Input: part model. Units: mm. Frame: model coordinates. Coordinates: 2 decimals unless noted, no trailing zeros. Order: outer loops, then holes, each group sorted by start corner. A loop starts at its lowest first (then second) coordinate and runs counter-clockwise, first axis right, second up. Notation, with made-up numbers: (70, 18) -> (94, 18) arc R15 ccw to (94, 25) -> close; hole circle Ø3 at (31, -6). An arc over 180 degrees is marked (long way). Use one line per item in the form item = value. Start each with the question number.
1) Pin query (flat end, axial travel): pin 1 (2.5 mm diameter, centred on y = 160.5, z = 3, fed in from +X) (3 decimals); pin 2 (1.5 mm diameter, centred on y = 41, z = 3, fed in from -X) (3 decimals); pin 3 (1.4 mm diameter, centred on x = 116, z = 3, fed in from +Y). Return the tip coordinate at first contact, or that it passes through.
2) Section query B-B on x = 100. Output: boundary loops of the cut face in (y, z), then the cut area to 3 significant figures.
3) Section query A-A on y = 130. Output: boundary loops of the cut face in (x, z).
4) Ray query, line 1 along X through (y, z) = (9.5, 0.4); line 2 along Y through (x, z) = (19, 0.35); line 3 along Y through (x, z) = (103, 1.05). Return the intervals inside material, ascending.
from build123d import *

# Parameters (mm, degrees)
BOSS_EXTRUDE1_DEPTH = 4.826
CUT_EXTRUDE1_DEPTH  = 283.027055929
SKETCH3_R           = 23.114
CUT_EXTRUDE2_DEPTH  = 4.826
SKETCH4_W           = 20.32
SKETCH4_H           = 4.617249963
CUT_EXTRUDE3_DEPTH  = 283.027055929
SKETCH5_W           = 20.32
SKETCH5_H           = 4.826
CUT_EXTRUDE4_DEPTH  = 283.027055929


with BuildPart() as part:
    # Sketch1 → Boss-Extrude1 (new body)
    with BuildSketch(Plane.XY):
        Polygon((228.6, 165.1), (0, 165.1), (82.55, 0), (146.05, 0), align=None)
    extrude(amount=BOSS_EXTRUDE1_DEPTH)

    # Sketch2 → Cut-Extrude1 (cut, through all)
    with BuildSketch(Plane.XY.offset(4.826)):
        Polygon((20.097936797, 124.904126406), (24.414442421, 127.062379218), (35.002974022, 105.885316015), (30.686468399, 103.727063203), align=None)
        Polygon((41.275, 82.55), (45.591505624, 84.708252812), (56.180037225, 63.531189609), (51.863531601, 61.372936797), align=None)
        Polygon((62.452063203, 40.195873594), (66.768568827, 42.354126406), (77.357100428, 21.177063203), (73.040594804, 19.018810391), align=None)
        Polygon((155.559405196, 19.018810391), (166.147936797, 40.195873594), (161.831431173, 42.354126406), (151.242899572, 21.177063203), align=None)
        Polygon((176.736468399, 61.372936797), (187.325, 82.55), (183.008494376, 84.708252812), (172.419962775, 63.531189609), align=None)
        Polygon((197.913531601, 103.727063203), (208.502063203, 124.904126406), (204.185557579, 127.062379218), (193.597025978, 105.885316015), align=None)
    extrude(amount=-CUT_EXTRUDE1_DEPTH, mode=Mode.SUBTRACT)

    # Sketch3 → Cut-Extrude2 (cut)
    with BuildSketch(Plane.XY.offset(4.826)):
        with Locations((114.3, -7.62)):
            Circle(SKETCH3_R)
    extrude(amount=-CUT_EXTRUDE2_DEPTH, mode=Mode.SUBTRACT)

    # Sketch4 → Cut-Extrude3 (cut, through all)
    with BuildSketch(Plane.XY.offset(4.826)):
        with Locations((154.974498273, 165.599419735)):
            Rectangle(SKETCH4_W, SKETCH4_H)
        with Locations((114.334498273, 165.599419735)):
            Rectangle(SKETCH4_W, SKETCH4_H)
        with Locations((73.694498273, 165.599419735)):
            Rectangle(SKETCH4_W, SKETCH4_H)
    extrude(amount=-CUT_EXTRUDE3_DEPTH, mode=Mode.SUBTRACT)

    # Sketch5 → Cut-Extrude4 (cut, through all)
    with BuildSketch(Plane.XY.offset(4.826)):
        with Locations((154.974498273, 160.877794753)):
            Rectangle(SKETCH5_W, SKETCH5_H)
        with Locations((114.334498273, 160.877794753)):
            Rectangle(SKETCH5_W, SKETCH5_H)
        with Locations((73.694498273, 160.877794753)):
            Rectangle(SKETCH5_W, SKETCH5_H)
    extrude(amount=-CUT_EXTRUDE4_DEPTH, mode=Mode.SUBTRACT)


solid = part.part
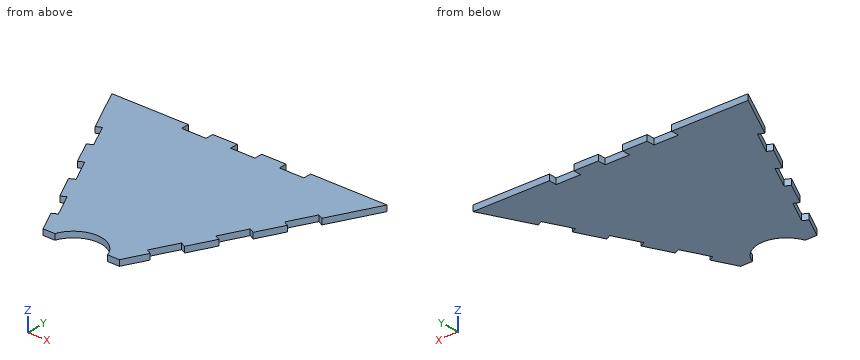
Answers below:
q1.pin_1 = 226.925
q1.pin_2 = 61.675
q1.pin_3 = 158.46
q2.outline = (10.54, 0) -> (165.1, 0) -> (165.1, 4.83) -> (10.54, 4.83) -> close
q2.area = 746 mm^2
q3.outline = (17.55, 0) -> (211.05, 0) -> (211.05, 4.83) -> (17.55, 4.83) -> close
q4.line_1 = 77.8 to 98.77, 129.83 to 150.8
q4.line_2 = 127.1 to 165.1
q4.line_3 = 12.54 to 165.1
